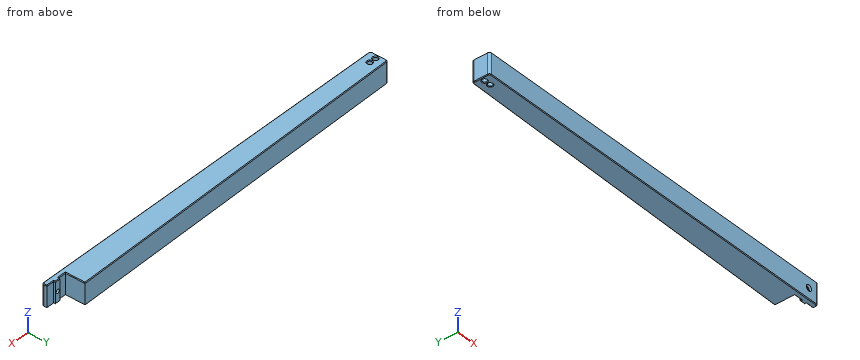
```python
from build123d import *

# Parameters (mm, degrees)
SKETCH1_R           = 2.05
BOSS_EXTRUDE1_DEPTH = 20
SKETCH2_R           = 1.7
CUT_EXTRUDE1_DEPTH  = 20
SKETCH3_R           = 2.8
CUT_EXTRUDE2_DEPTH  = 2
FILLET1_R           = 2
CHAMFER1_SIZE       = 0.6
CHAMFER2_SIZE       = 0.6


with BuildPart() as part:
    # Sketch1 → Boss-Extrude1 (new body)
    with BuildSketch(Plane.XY):
        Polygon((15.2, -92.57905153), (15.2, -76.05265525), (349.336279792, -69.740004959), (349.336279792, -87.940004959), (356.686279792, -87.940004959), (356.686279792, -86.440004959), (361.986279792, -86.440004959), (361.986279792, -87.940004959), (369.336279792, -87.940004959), (369.336279792, -92.57905153), align=None)
        with Locations((25.300294751, -84.31585339)):
            Circle(SKETCH1_R, mode=Mode.SUBTRACT)
        with Locations((19.300294751, -84.31585339)):
            Circle(SKETCH1_R, mode=Mode.SUBTRACT)
    extrude(amount=BOSS_EXTRUDE1_DEPTH)

    # Sketch2 → Cut-Extrude1 (cut)
    with BuildSketch(Plane(origin=(0, -92.57905153, 0), x_dir=(-1, 0, 0), z_dir=(0, -1, 0))):
        with Locations((-359.336279792, -10)):
            Circle(SKETCH2_R)
    extrude(amount=-CUT_EXTRUDE1_DEPTH, mode=Mode.SUBTRACT)

    # Sketch3 → Cut-Extrude2 (cut)
    with BuildSketch(Plane.XZ.offset(92.57905153)):
        with Locations((359.336279792, 10)):
            Circle(SKETCH3_R)
    extrude(amount=-CUT_EXTRUDE2_DEPTH, mode=Mode.SUBTRACT)

    # Fillet1
    fillet1_edges = [part.edges().sort_by_distance(p)[0] for p in [
        (15.2, -92.57905153, 10),
        (15.2, -76.05265525, 10),
        (369.336279792, -92.57905153, 10),
    ]]
    fillet(fillet1_edges, radius=FILLET1_R)

    # Chamfer1
    chamfer1_edges = [part.edges().sort_by_distance(p)[0] for p in [
        (183.249250825, -72.877794523, 0),
        (349.336279792, -78.840004959, 0),
        (353.011279792, -87.940004959, 0),
        (356.686279792, -87.190004959, 0),
        (359.336279792, -86.440004959, 0),
        (361.986279792, -87.190004959, 0),
        (365.661279792, -87.940004959, 0),
        (23.250294751, -84.31585339, 0),
        (17.250294751, -84.31585339, 0),
        (369.336279792, -89.259528244, 0),
        (192.268139896, -92.57905153, 0),
        (15.2, -84.297139394, 0),
        (15.785786438, -91.993265092, 0),
        (15.772492332, -76.614433962, 0),
        (368.750493354, -91.993265092, 0),
    ]]
    chamfer(chamfer1_edges, length=CHAMFER1_SIZE)

    # Chamfer2
    chamfer2_edges = [part.edges().sort_by_distance(p)[0] for p in [
        (365.661279792, -87.940004959, 20),
        (361.986279792, -87.190004959, 20),
        (359.336279792, -86.440004959, 20),
        (356.686279792, -87.190004959, 20),
        (23.250294751, -84.31585339, 20),
        (353.011279792, -87.940004959, 20),
        (17.250294751, -84.31585339, 20),
        (349.336279792, -78.840004959, 20),
        (183.249250825, -72.877794523, 20),
        (369.336279792, -89.259528244, 20),
        (192.268139896, -92.57905153, 20),
        (15.2, -84.297139394, 20),
        (15.785786438, -91.993265092, 20),
        (15.772492332, -76.614433962, 20),
        (368.750493354, -91.993265092, 20),
    ]]
    chamfer(chamfer2_edges, length=CHAMFER2_SIZE)


solid = part.part
```
Read the model definition and answer for the solid it produces. Units are mm, in the model's axes. Give positions to 0.01 mm unless a question says otherwise; leave off trailing zeros. Write each loop counter-clockwise with the first axis right and the second up, starting at its lowest first coordinate (ties: lowest second). Pieces come first, ordered by that corner, then holes. Notation, with made-up numbers: (5.25, -38) -> (54.25, -38) arc R11 cw to (54.25, -31) -> close; hole circle Ø9 at (41, -17). An arc over 180 degrees is marked (long way). Answer in a Markdown table with one row per item.
1) Section A-A on z = 16.5 is taken. Give the vertices of the cut face in (x, y).
Results list:
| item | result |
|---|---|
| outline | (15.2, -90.58) arc R2 ccw to (17.2, -92.58) -> (367.34, -92.58) arc R2 ccw to (369.34, -90.58) -> (369.34, -87.94) -> (361.99, -87.94) -> (361.99, -86.44) -> (356.69, -86.44) -> (356.69, -87.94) -> (349.34, -87.94) -> (349.34, -69.74) -> (17.16, -76.02) arc R2 ccw to (15.2, -78.02) -> close; hole circle Ø4.1 at (19.3, -84.32); hole circle Ø4.1 at (25.3, -84.32) |
2) Section B-B on x = 224 is taken. Give the vertices of the cut face in (y, z), plus the area to 3 significant figures.
Results list:
| item | result |
|---|---|
| outline | (-92.58, 0.6) -> (-91.98, 0) -> (-72.71, 0) -> (-72.11, 0.6) -> (-72.11, 19.4) -> (-72.71, 20) -> (-91.98, 20) -> (-92.58, 19.4) -> close |
| area | 409 mm^2 |
3) Straight lines are drawn through the part: line 1 (X direction, y = -84, z = 6); line 2 (X direction, y = -89.45, z = 10); line 3 (X direction, y = -87, z = 15.5). For each, find the intervals that lie inside material, in ascending order. Write a range as [from, to].
Results list:
| item | result |
|---|---|
| line 1 | [15.2, 17.27], [21.33, 23.27], [27.33, 349.34] |
| line 2 | [15.2, 357.64], [361.04, 369.34] |
| line 3 | [15.2, 349.34], [356.69, 361.99] |
4) Each of these flat-tipped pins is pushed along its axis until it touches: pin 1 Ø1.6 at (y, z) = (-87, 12.5) entering from +X; pin 2 Ø9 at (x, z) = (359.34, 10) entering from +Y; pin 3 Ø1.5 at (x, z) = (329, 12.5) entering from +Y. Where does it stop, or does it pass through?
Results list:
| item | result |
|---|---|
| pin 1 | x = 361.99 |
| pin 2 | y = -86.44 |
| pin 3 | y = -70.11 |
5) Section C-C on x = 40 is taken. Give the vertices of the cut face in (y, z), plus the area to 3 significant figures.
Results list:
| item | result |
|---|---|
| outline | (-92.58, 0.6) -> (-91.98, 0) -> (-76.18, 0) -> (-75.58, 0.6) -> (-75.58, 19.4) -> (-76.18, 20) -> (-91.98, 20) -> (-92.58, 19.4) -> close |
| area | 339 mm^2 |
